Work out the finished part from the listing and answer in its coordinate system (mm). A direction names the side the tool comes from. Give positions to 0.01 mm unless a question says otherwise; leave off trailing zeros. Loops run counter-clockwise (first coordinate to the right, second up) from the corner with the lowest first, then second, coordinate; pieces in that order, holes last.
```python
from build123d import *

# Parameters (mm, degrees)
SKETCH_R        = 35
PAD_DEPTH       = 5
SKETCH001_R     = 12.5
PAD001_DEPTH    = 80
SKETCH003_R     = 1.25
POCKET_DEPTH    = 35.001
SKETCH004_R     = 3.6
POCKET001_DEPTH = 85.001
SKETCH005_R     = 4.25
HOLE_DEPTH      = 55
HOLE_TIPS_R     = 4.25
CHAMFER_SIZE    = 1
SKETCH006_W     = 25.864929
SKETCH006_H     = 80.956299
POCKET002_DEPTH = 5.001


with BuildPart() as part:
    # Sketch → Pad (new body)
    with BuildSketch(Plane.XY):
        Circle(SKETCH_R)
    extrude(amount=PAD_DEPTH)

    # Sketch001 (on Face3 of Pad) → Pad001 (join)
    with BuildSketch(Plane.XY.offset(5)):
        Circle(SKETCH001_R)
    extrude(amount=PAD001_DEPTH)

    # Sketch002 (on DatumPlane) → Groove (revolve, cut)
    with BuildSketch(Plane.XZ):
        with BuildLine():
            Line((10.5, 68.999986), (10.5, 20.999986))
            ThreePointArc((10.5, 20.999986), (11.232238, 19.232228), (13, 18.5))
            Line((13, 71.5), (13, 18.5))
            ThreePointArc((13, 71.5), (11.232228, 70.767762), (10.5, 68.999986))
        make_face()
    revolve(axis=Axis((13, 0, 0), (0, 0, -1)), mode=Mode.SUBTRACT)

    # Sketch003 (on DatumPlane) → Pocket (cut, through all)
    with BuildSketch(Plane.YZ):
        with Locations((0, 45)):
            Circle(SKETCH003_R)
    extrude(amount=POCKET_DEPTH, mode=Mode.SUBTRACT)

    # Sketch004 (on Face2 of Pocket) → Pocket001 (cut, through all)
    with BuildSketch(Plane(origin=(0, 0, 0), x_dir=(1, 0, 0), z_dir=(0, 0, -1))):
        with Locations((25, 0)):
            Circle(SKETCH004_R)
    extrude(amount=-POCKET001_DEPTH, mode=Mode.SUBTRACT)

    # Sketch005 (on Face2 of Pocket001) → Hole (cut)
    with BuildSketch(Plane(origin=(0, 0, 0), x_dir=(1, 0, 0), z_dir=(0, 0, -1))):
        Circle(SKETCH005_R)
    extrude(amount=-HOLE_DEPTH, mode=Mode.SUBTRACT)

    # Hole tips → Hole tip 1 section 0
    with BuildSketch(Plane(origin=(0, 0, 55), x_dir=(1, 0, 0), z_dir=(0, 0, -1)), mode=Mode.PRIVATE) as hole_tip_1_s0:
        Circle(HOLE_TIPS_R)
    loft([hole_tip_1_s0.sketch, Vertex(0, 0, 57.553658)], mode=Mode.SUBTRACT)

    # Chamfer
    chamfer_edges = [part.edges().sort_by_distance(p)[0] for p in [
        (-12.5, 0, 85),
    ]]
    chamfer(chamfer_edges, length=CHAMFER_SIZE)

    # Sketch006 (on Face9 of Clone) → Pocket002 (cut, through all)
    with BuildSketch(Plane.XY.offset(5)):
        with Locations((-32.932464, -3.256923)):
            Rectangle(SKETCH006_W, SKETCH006_H)
    extrude(amount=-POCKET002_DEPTH, mode=Mode.SUBTRACT)


solid = part.part
```
Q1. Consider line 1 along X through (y, z) = (0, 3); line 2 along Z through (x, y) = (9, 0); line 3 along Z through (x, y) = (13, 28). Determine where each line is inside the solid, lowest interval first.
Q2. Determine the mould class of faces 4 (the face through (21.403, -0.158, 2.465)), 5 (the face through (13, 0, 5)), 6 (the face through (11.923, 3.755, 43.947)) for opening direction Y: +Y half, -Y half, draft (parallel to the pull), parting line (faces both ways), or undercut.
Q3. Given pin 1 (3 mm diameter, centred on x = 23.5, y = 13, fed in from +Z); pin 2 (4 mm diameter, centred on y = -13, z = 23.5, fed in from -X); pin 3 (6 mm diameter, centred on y = -12.5, z = 24.5, fed in from +X); pin 4 (12 mm diameter, centred on x = 27.5, y = -1.5, fed in from -Z), each flat-ended and moving along its own axis, determine where each tip first touches the part or whether it passes through.
Q4. Section C-C on z = 45 is taken. Give the vertices of the cut face in (x, y).
Q5. Section B-B on z = 31.5 is taken. Give the vertices of the cut face in (x, y).
Q6. Section D-D on y = 13.5 is taken. Give the vertices of the cut face in (x, z), plus the area to 3 significant figures.
Q7. Which of the six approach directions +Z, -Z, +X, -X, +Y, -Y give full straight-line access (tool end or side, diameter ignored) to faces 1 (the face through (2.285, -3.584, 27.115)), 2 (the face through (7.4, -0.16, 46.24)), 3 (the face through (34.984, -1.068, 2.465))?
Q8. Section A-A on x = 25 is taken. Give the vertices of the cut face in (y, z).
Check result:
1. line 1: x = -20 to -4.25, 4.25 to 21.4, 28.6 to 35
1. line 2: z = 0 to 43.75, 46.25 to 85
1. line 3: z = 0 to 5
2. face 4: undercut
2. face 5: draft
2. face 6: parting line
3. pin 1: stops at z = 5
3. pin 2: stops at x = -5.94
3. pin 3: stops at x = 8.12
3. pin 4: stops at z = 0
4. outline: (4.06, -1.25) arc R4.25 cw (long way) to (4.06, 1.25) - (10.83, 1.25) arc R2.5 cw to (12.27, 2.39) arc R12.5 ccw (long way) to (12.27, -2.39) arc R2.5 cw to (10.83, -1.25) - close
5. outline: (12.27, -2.39) arc R2.5 cw to (12.27, 2.39) arc R12.5 ccw (long way) to start; hole circle Ø8.5 at (0, 0)
6. outline: (-20, 0) - (32.29, 0) - (32.29, 5) - (-20, 5) - close
6. area: 261 mm2
7. face 1: -Z
7. face 2: +X
7. face 3: +Z, -Z
8. outline: (-24.49, 0) - (-3.6, 0) - (-3.6, 5) - (-24.49, 5) - close; (3.6, 0) - (24.49, 0) - (24.49, 5) - (3.6, 5) - close
